from build123d import *

# Parameters (mm, degrees)
CROQUIS1_R              = 11.5
SALIENTE_EXTRUIR1_DEPTH = 5
CROQUIS2_R              = 4.99
SALIENTE_EXTRUIR2_DEPTH = 5
CROQUIS3_R              = 1.6
CORTAR_EXTRUIR1_DEPTH   = 6
CORTAR_EXTRUIR2_DEPTH   = 11
CROQUIS5_R              = 3.1
CORTAR_EXTRUIR3_DEPTH   = 3.5


with BuildPart() as part:
    # Croquis1 → Saliente-Extruir1 (new body)
    with BuildSketch(Plane(origin=(0, 0, 0), x_dir=(1, 0, 0), z_dir=(0, 1, 0))):
        Circle(CROQUIS1_R)
    extrude(amount=SALIENTE_EXTRUIR1_DEPTH)

    # Croquis2 → Saliente-Extruir2 (add)
    with BuildSketch(Plane.XZ):
        Circle(CROQUIS2_R)
    extrude(amount=SALIENTE_EXTRUIR2_DEPTH)

    # Croquis3 → Cortar-Extruir1 (cut, through all)
    with BuildSketch(Plane.XZ):
        with Locations((-8.245, 0)):
            Circle(CROQUIS3_R)
        with Locations((8.245, 0)):
            Circle(CROQUIS3_R)
    extrude(amount=-CORTAR_EXTRUIR1_DEPTH, mode=Mode.SUBTRACT)

    # Croquis4 → Cortar-Extruir2 (cut, through all)
    with BuildSketch(Plane.XZ.offset(5)):
        with BuildLine():
            Line((-1.55, 2.024845673), (-1.55, -2.024845673))
            ThreePointArc((-1.55, -2.024845673), (2.55, 0), (-1.55, 2.024845673))
        make_face()
    extrude(amount=-CORTAR_EXTRUIR2_DEPTH, mode=Mode.SUBTRACT)

    # Croquis5 → Cortar-Extruir3 (cut)
    with BuildSketch(Plane(origin=(0, 5, 0), x_dir=(1, 0, 0), z_dir=(0, 1, 0))):
        with Locations((-8.245, 0)):
            Circle(CROQUIS5_R)
        with Locations((8.245, 0)):
            Circle(CROQUIS5_R)
    extrude(amount=-CORTAR_EXTRUIR3_DEPTH, mode=Mode.SUBTRACT)


solid = part.part
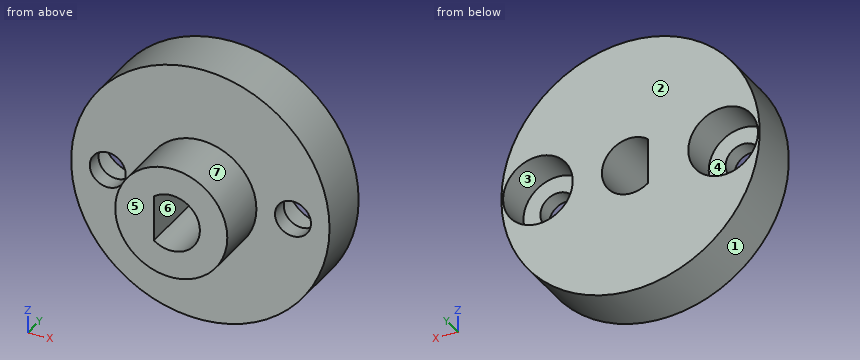
Geometry: final body of the model. Coordinates: model frame, mm. Face numbers are marked on the shaded views. A direction names the side the tool comes from. Give positions to 0.01 mm unless a question says otherwise; leave off trailing zeros. Write each loop counter-clockwise with the first axis right and the second up, starting at its lowest first coordinate (ties: lowest second). Pieces come first, ordered by that corner, then holes. Notation, with made-up numbers: (33.5, 63.5) - (84.5, 63.5) arc R31 ccw to (84.5, 100.5) - close; hole circle Ø1 at (62.25, 59.25). An arc over 180 degrees is marked (long way). Return JSON: item names as keys, results as strings. Group by question number.
1) Line query: line 1 (X direction, y = 3.7, z = 0) (3 decimals); line 2 (Y direction, x = -5, z = 5.75); line 3 (Y direction, x = 5.5, z = -1). Output: solid intervals per line, ascending.
2) First-contact query: P1, Ø1, axis at x = 3.5, y = 2.5, coming from the +Z side; P2, Ø5, axis at x = -8.245, z = 0, coming from the +Y side; P3, Ø1, axis at y = 1, z = -5.5, coming from the +X side; P4, Ø7, axis at x = -8.245, z = 0, coming from the +Y side. Flat tips, straight axial feed; report the tip coordinate or a pass-through.
3) Section B-B on x = 0. Return the cut outline in (y, z).
4) Section D-D on x = -5.75. Return the cut outline in (y, z).
5) Section A-A on z = 0. Return the cut outline in (x, y) (3 decimals).
6) Section C-C on y = 3.75. Return the cut outline in (x, z) (3 decimals).
7) Set-up query: the marked faces 4, 5, 6 and 7. Return all of +Z, -Z, +X, -X, +Y, -Y with unobstructed straight access to the full face (end or side cutting, diameter ignored); none if empty.
8) Mould query, pull axis Z, two halves, no side actions, for the marked faces 1, 2 and 3. Classes: released by +Z, released by -Z, zero draft, split by the parting line, or undercut.
Filled in:
{
 "1": {"line 1": "x = -11.5 to -11.345, -5.145 to -1.55, 2.55 to 5.145, 11.345 to 11.5", "line 2": "y = 0 to 5", "line 3": "y = 0 to 1.5"},
 "2": {"P1": "stops at z = 11.1", "P2": "stops at y = 1.5", "P3": "stops at x = 10.36", "P4": "stops at y = 5"},
 "3": {"outline": "(-5, -4.99) - (0, -4.99) - (0, -11.5) - (5, -11.5) - (5, -2.55) - (-5, -2.55) - close; (-5, 2.55) - (5, 2.55) - (5, 11.5) - (0, 11.5) - (0, 4.99) - (-5, 4.99) - close"},
 "4": {"outline": "(0, -9.96) - (5, -9.96) - (5, -1.84) - (1.5, -1.84) - (1.5, 1.84) - (5, 1.84) - (5, 9.96) - (0, 9.96) - close"},
 "5": {"outline": "(-11.5, 0) - (-9.845, 0) - (-9.845, 1.5) - (-11.345, 1.5) - (-11.345, 5) - (-11.5, 5) - close; (-6.645, 0) - (-4.99, 0) - (-4.99, -5) - (-1.55, -5) - (-1.55, 5) - (-5.145, 5) - (-5.145, 1.5) - (-6.645, 1.5) - close; (2.55, -5) - (4.99, -5) - (4.99, 0) - (6.645, 0) - (6.645, 1.5) - (5.145, 1.5) - (5.145, 5) - (2.55, 5) - close; (9.845, 0) - (11.5, 0) - (11.5, 5) - (11.345, 5) - (11.345, 1.5) - (9.845, 1.5) - close"},
 "6": {"outline": "circle Ø23 at (0, 0); hole circle Ø6.2 at (-8.245, 0); hole (-1.55, -2.025) arc R2.55 ccw (long way) to (-1.55, 2.025) - close; hole circle Ø6.2 at (8.245, 0)"},
 "7": {"face 4": "+Y", "face 5": "+Z, -Z, +X, -X, -Y", "face 6": "+Y, -Y", "face 7": "-Y"},
 "8": {"face 1": "split by the parting line", "face 2": "zero draft", "face 3": "undercut"}
}
